```python
from build123d import *

# Parameters (mm, degrees)
SKETCH1_W               = 63.5
SKETCH1_H               = 50.8
BOSS_EXTRUDE1_DEPTH     = 12.7
CUT_EXTRUDE1_START      = -5.588
SKETCH2_R               = 7.493
CUT_EXTRUDE1_DEPTH      = 5.588
CUT_EXTRUDE2_START      = -5.588
SKETCH3_W               = 31.75
SKETCH3_H               = 1.778
CUT_EXTRUDE2_DEPTH      = 5.588
SKETCH9_R               = 1.9939
CUT_EXTRUDE3_DEPTH      = 11.9888
CUT_EXTRUDE4_START      = -4.572
SKETCH10_R              = 7.493
CUT_EXTRUDE4_DEPTH      = 4.572
SKETCH11_R              = 2.5527
CUT_EXTRUDE5_DEPTH      = 13.7
MIRROR2_COPY_1_SKETCH_R = 2.5527
MIRROR2_COPY_1_DEPTH    = 13.7


with BuildPart() as part:
    # Sketch1 → Boss-Extrude1 (new body)
    with BuildSketch(Plane.XY):
        Rectangle(SKETCH1_W, SKETCH1_H)
    extrude(amount=BOSS_EXTRUDE1_DEPTH)

    # Sketch2 → Cut-Extrude1 (cut)
    with BuildSketch(Plane.XY.offset(12.7).offset(CUT_EXTRUDE1_START)):
        with Locations((-5.08, 0)):
            Circle(SKETCH2_R)
    extrude(amount=CUT_EXTRUDE1_DEPTH, mode=Mode.SUBTRACT)

    # Sketch3 → Cut-Extrude2 (cut)
    with BuildSketch(Plane.XY.offset(12.7).offset(CUT_EXTRUDE2_START)):
        with Locations((15.875, 0)):
            Rectangle(SKETCH3_W, SKETCH3_H)
    extrude(amount=CUT_EXTRUDE2_DEPTH, mode=Mode.SUBTRACT)

    # Sketch9 → Cut-Extrude3 (cut)
    with BuildSketch(Plane.XY.offset(7.112)):
        with Locations((-5.08, 0)):
            Circle(SKETCH9_R)
    extrude(amount=-CUT_EXTRUDE3_DEPTH, mode=Mode.SUBTRACT)

    # Sketch10 → Cut-Extrude4 (cut)
    with BuildSketch(Plane(origin=(0, 0, 0), x_dir=(-1, 0, 0), z_dir=(0, 0, -1)).offset(CUT_EXTRUDE4_START)):
        with Locations((5.08, 0)):
            Circle(SKETCH10_R)
    extrude(amount=CUT_EXTRUDE4_DEPTH, mode=Mode.SUBTRACT)

    # Sketch11 → Cut-Extrude5 (cut, through all)
    with BuildSketch(Plane.XY.offset(12.7)):
        with Locations((-25.4, 19.05)):
            Circle(SKETCH11_R)
    cut_extrude5 = extrude(amount=-CUT_EXTRUDE5_DEPTH, mode=Mode.SUBTRACT)

    # Mirror1: Cut-Extrude5 across plane
    add(cut_extrude5.mirror(Plane(origin=(0, 0, 0), x_dir=(0, 0, 1), z_dir=(1, 0, 0))), mode=Mode.SUBTRACT)

    # Mirror2: Cut-Extrude5 across plane
    add(cut_extrude5.mirror(Plane.ZX), mode=Mode.SUBTRACT)

    # Mirror2 copy 1 sketch → Mirror2 copy 1 (cut, through all)
    with BuildSketch(Plane(origin=(0, 0, 12.7), x_dir=(-1, 0, 0), z_dir=(0, 0, 1))):
        with Locations((-25.4, 19.05)):
            Circle(MIRROR2_COPY_1_SKETCH_R)
    extrude(amount=-MIRROR2_COPY_1_DEPTH, mode=Mode.SUBTRACT)


solid = part.part
```
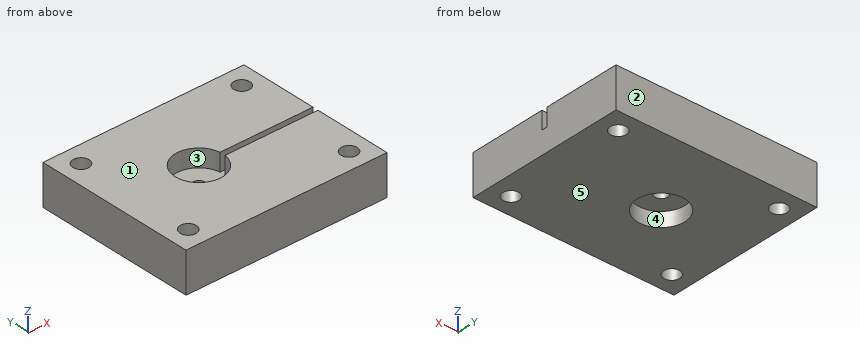
Verification items for the finished model (mm, model axes). Face numbers are marked on the shaded views. A direction names the side the tool comes from. Round coordinates to 2 decimals unless told otherwise and drop trailing zeros. Write each loop counter-clockwise with the first axis right and the second up, starting at its lowest first coordinate (ties: lowest second). Pieces come first, ordered by that corner, then holes.
1. Section check B-B on x = 25.4. Enter the section's corners in (y, z).
2. Section check A-A on y = -19.05. Enter the section's corners in (x, z), plus the area to 3 significant figures.
3. Scan lines: L1, parallel to Y at x = -25.4, z = 7.5; L2, parallel to Y at x = 21, z = 10; L3, parallel to Y at x = -5.08, z = 9.7. Record each from-to range of solid material in increasing order.
4. Draft check along Y on the marked faces 1, 2 and 3. Enter one of: +Y half, -Y half, draft (parallel to the pull), parting line (faces both ways), or undercut.
5. Access from +Z, -Z, +X, -X, +Y, -Y to the whole of each face (thin tool, end or side, straight path). Record for the marked faces 4 and 5.
6. Section check D-D on x = -5.08. Enter the section's corners in (y, z), plus the area to 3 significant figures.
7. Gauge pin test, flat ends, axial feed: P1, Ø6.5, axis at x = -5.08, y = 0, coming from the +Z side; P2, Ø3, axis at x = 25.4, y = -19.05, coming from the +Z side. Record the tip position at first contact, or that the pin passes through.
8. Section check C-C on z = 5.5. Enter the section's corners in (x, y), plus the area to 3 significant figures.
Answer:
1. outline: (-25.4, 0) - (-21.6, 0) - (-21.6, 12.7) - (-25.4, 12.7) - close; (-16.5, 0) - (16.5, 0) - (16.5, 12.7) - (0.89, 12.7) - (0.89, 7.11) - (-0.89, 7.11) - (-0.89, 12.7) - (-16.5, 12.7) - close; (21.6, 0) - (25.4, 0) - (25.4, 12.7) - (21.6, 12.7) - close
2. outline: (-31.75, 0) - (-27.95, 0) - (-27.95, 12.7) - (-31.75, 12.7) - close; (-22.85, 0) - (22.85, 0) - (22.85, 12.7) - (-22.85, 12.7) - close; (27.95, 0) - (31.75, 0) - (31.75, 12.7) - (27.95, 12.7) - close
2. area: 677 mm2
3. L1: y = -25.4 to -21.6, -16.5 to 16.5, 21.6 to 25.4
3. L2: y = -25.4 to -0.89, 0.89 to 25.4
3. L3: y = -25.4 to -7.49, 7.49 to 25.4
4. face 1: draft
4. face 2: +Y half
4. face 3: undercut
5. face 4: -Z
5. face 5: -Z, +X, -X, +Y, -Y
6. outline: (-25.4, 0) - (-7.49, 0) - (-7.49, 4.57) - (-1.99, 4.57) - (-1.99, 7.11) - (-7.49, 7.11) - (-7.49, 12.7) - (-25.4, 12.7) - close; (1.99, 4.57) - (7.49, 4.57) - (7.49, 0) - (25.4, 0) - (25.4, 12.7) - (7.49, 12.7) - (7.49, 7.11) - (1.99, 7.11) - close
6. area: 483 mm2
7. P1: stops at z = 7.11
7. P2: passes through
8. outline: (-31.75, -25.4) - (31.75, -25.4) - (31.75, 25.4) - (-31.75, 25.4) - close; hole circle Ø5.11 at (-25.4, -19.05); hole circle Ø5.11 at (-25.4, 19.05); hole circle Ø3.99 at (-5.08, 0); hole circle Ø5.11 at (25.4, -19.05); hole circle Ø5.11 at (25.4, 19.05)
8. area: 3,130 mm2
